The model under review builds one solid part; all positions refer to its coordinate system, in mm. A direction names the side the tool comes from. Coordinates: 2 decimals unless noted, no trailing zeros. Write each loop counter-clockwise with the first axis right and the second up, starting at its lowest first coordinate (ties: lowest second). Pieces come first, ordered by that corner, then holes.
```python
from build123d import *

# Parameters (mm, degrees)
SKETCH1_W                = 20
SKETCH1_H                = 16
SKETCH1_W_2              = 12.5
SKETCH1_H_2              = 10
BOSS_EXTRUDE1_DEPTH      = 170
FILLET1_R                = 4
FILLET2_R                = 4
SKETCH5_R                = 1
CUT_EXTRUDE2_DEPTH       = 21
BOSS_EXTRUDE2_DEPTH      = 4
BOSS_EXTRUDE2_DEPTH_BACK = 4
SKETCH7_W                = 13.8
SKETCH7_H                = 20
BOSS_EXTRUDE3_DEPTH      = 3.9
SKETCH8_R                = 1
CUT_EXTRUDE3_DEPTH       = 17.9
CUT_EXTRUDE4_DEPTH       = 21
SKETCH10_W               = 9
SKETCH10_H               = 14
BOSS_EXTRUDE4_DEPTH      = 4.5
SKETCH11_W               = 5.2
SKETCH11_H               = 3.2
CUT_EXTRUDE5_DEPTH       = 18.353591788
SKETCH12_W               = 1.641339812
SKETCH12_H               = 6.707183576
BOSS_EXTRUDE5_DEPTH      = 2


with BuildPart() as part:
    # Sketch1 → Boss-Extrude1 (new body)
    with BuildSketch(Plane.XY):
        Rectangle(SKETCH1_W, SKETCH1_H)
        Rectangle(SKETCH1_W_2, SKETCH1_H_2, mode=Mode.SUBTRACT)
    extrude(amount=BOSS_EXTRUDE1_DEPTH)

    # Fillet1
    fillet1_edges = [part.edges().sort_by_distance(p)[0] for p in [
        (10, -8, 85),
        (-10, -8, 85),
        (-10, 8, 85),
        (10, 8, 85),
    ]]
    fillet(fillet1_edges, radius=FILLET1_R)

    # Fillet2
    fillet2_edges = [part.edges().sort_by_distance(p)[0] for p in [
        (-6.25, 5, 85),
        (-6.25, -5, 85),
        (6.25, -5, 85),
        (6.25, 5, 85),
    ]]
    fillet(fillet2_edges, radius=FILLET2_R)

    # Sketch5 → Cut-Extrude2 (cut, through all)
    with BuildSketch(Plane.ZY.offset(10)):
        with Locations(Location((140, 0, 0), (0, 0, 270))):  # turned: the seam where the file's is
            Circle(SKETCH5_R)
    extrude(amount=-CUT_EXTRUDE2_DEPTH, mode=Mode.SUBTRACT)

    # Sketch6 → Boss-Extrude2 (add, two sides)
    with BuildSketch(Plane(origin=(0, 0, 0), x_dir=(0, 0, -1), z_dir=(1, 0, 0))) as boss_extrude2_sk:
        Polygon((0, 8), (-20.518331963, 8), (-19.805361375, 14.783462019), (0, 12), align=None)
    extrude(amount=BOSS_EXTRUDE2_DEPTH)
    extrude(boss_extrude2_sk.sketch, amount=-BOSS_EXTRUDE2_DEPTH_BACK)

    # Sketch7 → Boss-Extrude3 (add)
    with BuildSketch(Plane(origin=(0, 11.767570176, -1.653824135), x_dir=(1, 0, 0), z_dir=(0, 0.990268069, -0.139173101))):
        with Locations((0, -11.670077212)):
            Rectangle(SKETCH7_W, SKETCH7_H)
    extrude(amount=BOSS_EXTRUDE3_DEPTH)

    # Sketch8 → Cut-Extrude3 (cut, through all)
    with BuildSketch(Plane.ZY.offset(6.9)):
        with Locations(Location((10.181026889, 11.411194872, 0), (0, 0, 180))):  # turned: the seam where the file's is
            Circle(SKETCH8_R)
    extrude(amount=-CUT_EXTRUDE3_DEPTH, mode=Mode.SUBTRACT)

    # Sketch9 → Cut-Extrude4 (cut, through all)
    with BuildSketch(Plane(origin=(10, 0, 0), x_dir=(0, 0, -1), z_dir=(1, 0, 0))):
        Polygon((0.542775094, 15.862045468), (-3.375840567, -12.020353756), (9.67259421, -8.835863415), (6.237624145, 16.663737896), align=None)
    extrude(amount=-CUT_EXTRUDE4_DEPTH, mode=Mode.SUBTRACT)

    # Sketch10 → Boss-Extrude4 (add)
    with BuildSketch(Plane.XZ.offset(8)):
        with Locations((0, 9.810816694)):
            Rectangle(SKETCH10_W, SKETCH10_H)
    extrude(amount=BOSS_EXTRUDE4_DEPTH)

    # Sketch11 → Cut-Extrude5 (cut, through all)
    with BuildSketch(Plane.XY.offset(16.810816694)):
        with Locations((0, -9.6)):
            Rectangle(SKETCH11_W, SKETCH11_H)
    extrude(amount=-CUT_EXTRUDE5_DEPTH, mode=Mode.SUBTRACT)

    # Sketch12 → Boss-Extrude5 (add)
    with BuildSketch(Plane.XZ.offset(12.5)):
        with Locations((0, 2.810816694)):
            Rectangle(SKETCH12_W, SKETCH12_H)
    extrude(amount=BOSS_EXTRUDE5_DEPTH)


solid = part.part
```
Item 1: Take a section at A-A, the plane y = -9.5. Write out the cut boundary in (x, z), plus the area to 3 significant figures.
Solved:
outline: (-4.5, 2.81) - (-2.6, 2.81) - (-2.6, 16.81) - (-4.5, 16.81) - close; (2.6, 2.81) - (4.5, 2.81) - (4.5, 16.81) - (2.6, 16.81) - close
area: 53.2 mm2
Item 2: Mouldability with a two-part tool opening along Y and no side actions: class faces 6 (the face through (-0.1, 5.4, 170)), 7 (the face through (-0.097, 17.234, 9.221)), 8 (the face through (-8.859, -6.797, 87.299)), 9 (the face through (5.047, -3.859, 87.091)) as pulls with the +Y half, pulls with the -Y half, needs draft (parallel to the pull), parting line crosses it, or undercut.
Solved:
face 6: needs draft
face 7: pulls with the +Y half
face 8: pulls with the -Y half
face 9: undercut
Item 3: Machinability: for faces 1 (the face through (-5.47, 13.37, 9.76)), 2 (the face through (-5.047, 3.859, 86.675)), 3 (the face through (4.5, -10, 10)), 4 (the face through (6.9, 15, 10)), 5 (the face through (-6.9, 15, 10)), which of the approach directions +Z, -Z, +X, -X, +Y, -Y give a long, thin tool a straight path to every point of the face, cutting with its end or side? Answer none if there is none.
Solved:
face 1: +Z, -X
face 2: +Z, -Z
face 3: +Z, -Z, +X, -Y
face 4: +Z, -Z, +X, +Y
face 5: +Z, -Z, -X, +Y
Item 4: For pin 1 (1.6 mm diameter, centred on y = -10, z = 12, fed in from +X); pin 2 (1.4 mm diameter, centred on x = -1, z = 74.5, fed in from -Y); pin 3 (1.3 mm diameter, centred on y = -10, z = 7, fed in from -X), all flat-tipped, find the tip position at first contact; note any pin that passes through.
Solved:
pin 1: stops at x = 4.5
pin 2: stops at y = -8
pin 3: stops at x = -4.5
Item 5: To check wall thickness, follow line 1 along X through (y, z) = (0.5, 67); line 2 along Y through (x, z) = (-2, 68.5); line 3 along X through (y, z) = (-1.5, 106.5). State the ranges of each line that lie inside material, in increasing order.
Solved:
line 1: x = -10 to -6.25, 6.25 to 10
line 2: y = -8 to -5, 5 to 8
line 3: x = -10 to -6.22, 6.22 to 10
Item 6: Take a section at B-B, the plane z = 120. Write out the cut boundary in (x, y), plus the area to 3 significant figures.
Solved:
outline: (-10, -4) arc R4 ccw to (-6, -8) - (6, -8) arc R4 ccw to (10, -4) - (10, 4) arc R4 ccw to (6, 8) - (-6, 8) arc R4 ccw to (-10, 4) - close; hole (-6.25, -1) arc R4 ccw to (-2.25, -5) - (2.25, -5) arc R4 ccw to (6.25, -1) - (6.25, 1) arc R4 ccw to (2.25, 5) - (-2.25, 5) arc R4 ccw to (-6.25, 1) - close
area: 195 mm2
